The drawing under review shows one solid part. Ordinate dimensions are in mm from its lowest x, y, z. Coordinates: 2 decimals unless noted, no trailing zeros.
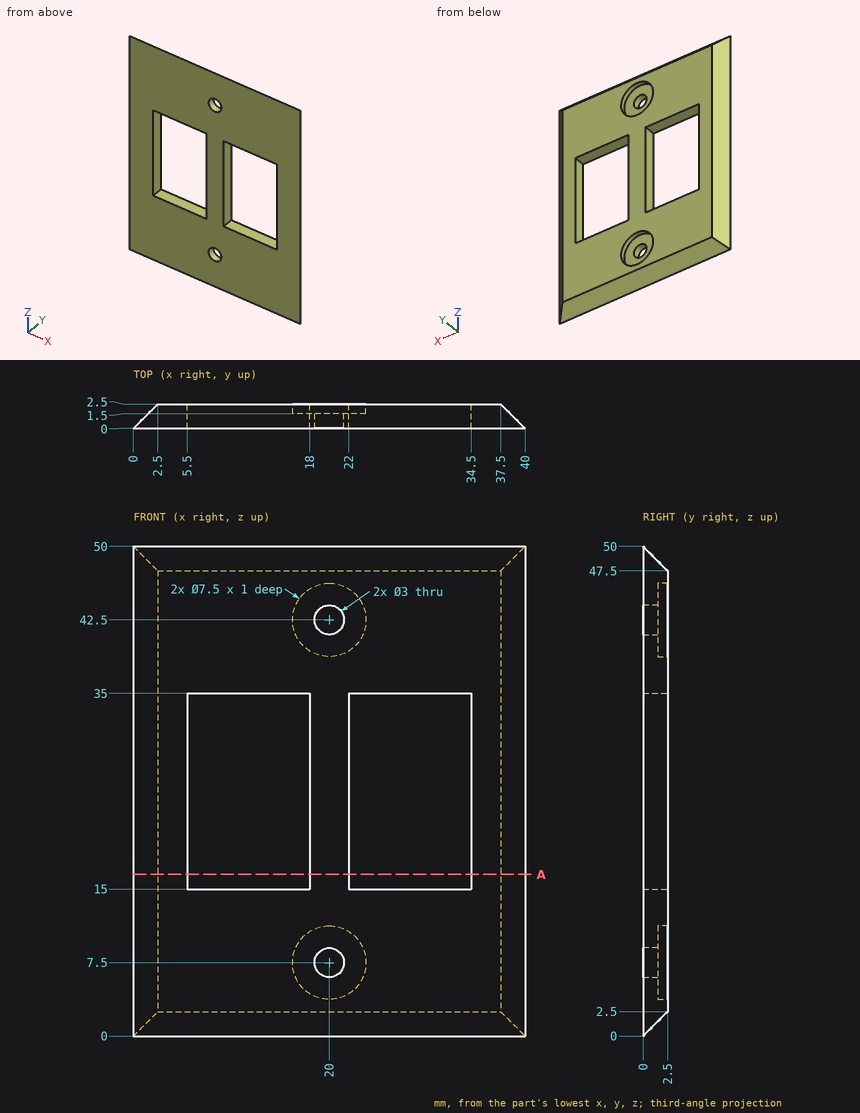
1) Consider section A-A (z = 16.5). Count the separate pieces of the cut face and the enclosed holes in it.
2) Clearance check with flat-ended pins moving along their axes: P1, Ø1.5, axis at x = 17.5, z = 19.5, coming from the +Y side; P2, Ø4, axis at x = 20, z = 42.5, coming from the +Y side; P3, Ø1.2, axis at x = 28.5, y = 1, coming from the -Z side; P4, Ø1.2, axis at y = 1.5, z = 21, coming from the -X side. State where each tip first meets the part, or that it passes through.
3) For L1, parallel to X at y = 1.6, z = 19.5; L2, parallel to X at y = 1.45, z = 21; L3, parallel to X at y = 1, z = 7.5, list the stretches that pass through material, from the lowest coordinate up.
Results:
1. separate pieces: 3
1. enclosed holes: 0
2. P1: stops at y = 2.5
2. P2: stops at y = 1.5
2. P3: stops at z = 0.4
2. P4: stops at x = 0.9
3. L1: x = 1.6 to 5.5, 18 to 22, 34.5 to 38.4
3. L2: x = 1.45 to 5.5, 18 to 22, 34.5 to 38.55
3. L3: x = 1 to 18.5, 21.5 to 39
